Source: CAD feature listing. Evaluate the final solid. Frame: model axes, mm. Coordinates: 2 decimals unless noted, no trailing zeros. Write each loop counter-clockwise with the first axis right and the second up, starting at its lowest first coordinate (ties: lowest second). Pieces come first, ordered by that corner, then holes. Notation, with made-up numbers: M -20.5,-21 L 6.5,-21 A23 cw 6.5,12 Z; hole C -28,55 d7. An arc over 180 degrees is marked long. One line per item, written item: value. Start each with the question number.
Item 1: Ray query, L1, parallel to Z at x = 80, y = 1.75 (3 decimals); L2, parallel to X at y = 1, z = -0.25; L3, parallel to X at y = 2.35, z = 10. Return the intervals inside material, ascending. Write a range as from..to.
Item 2: Cut plane C-C, the plane y = 0.45. State how many separate pieces and enclosed holes the cut face has, then the cut area to 3 significant figures.
Item 3: Cut plane B-B, the plane x = 0. Output: boundary loops of the cut face in (y, z) (3 decimals), then the cut area to 4 significant figures.
Item 4: Cut plane A-A, the plane z = 0. Output: boundary loops of the cut face in (x, y) (3 decimals), then the cut area to 3 significant figures.
Item 5: Pin query (flat end, axial travel): P1, Ø3, axis at x = 80, z = 0, coming from the +Y side; P2, Ø1.5, axis at x = 66.5, y = 0.5, coming from the -Z side. Return the tip coordinate at first contact, or that it passes through.
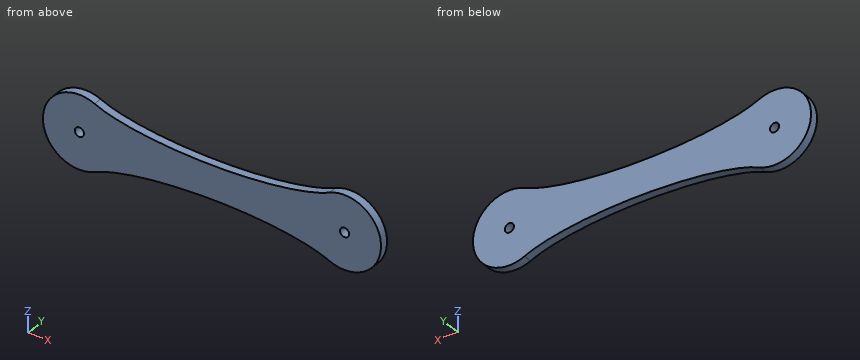
```python
from build123d import *

# Parameters (mm, degrees)
BOSS_EXTRUDE1_DEPTH = 2.6
CUT_EXTRUDE1_REACH  = 93.699
SKETCH3_R           = 1.375


with BuildPart() as part:
    # Sketch1 → Boss-Extrude1 (new body)
    with BuildSketch(Plane(origin=(0, 0, 0), x_dir=(1, 0, 0), z_dir=(0, 1, 0))):
        with BuildLine():
            ThreePointArc((4.582575695, 10), (-11, 0), (4.582575695, -10))
            add(Edge.make_bspline(
                [(4.582575695, -10), (11.56314995, -6.801099008), (40.099315353, -3.216443036), (68.360107676, -6.765931234), (75.417424305, -10)],
                knots=[0, 0, 0, 0, 0.499463492, 1, 1, 1, 1], degree=3))
            ThreePointArc((75.417424305, -10), (91, 0), (75.417424305, 10))
            add(Edge.make_bspline(
                [(4.582575695, 10), (11.56314995, 6.801099008), (40.099315353, 3.216443036), (68.360107676, 6.765931234), (75.417424305, 10)],
                knots=[0, 0, 0, 0, 0.499463492, 1, 1, 1, 1], degree=3))
        make_face()
    extrude(amount=BOSS_EXTRUDE1_DEPTH)

    # Sketch3 → Cut-Extrude1 (cut, up to next)
    with BuildSketch(Plane(origin=(0, 2.6, 0), x_dir=(1, 0, 0), z_dir=(0, 1, 0)), mode=Mode.PRIVATE) as cut_extrude1_sk1:
        with Locations(Location((0, 0, 0), (0, 0, 270))):
            Circle(SKETCH3_R)
    cut_extrude1_tool1 = extrude(cut_extrude1_sk1.sketch, amount=-CUT_EXTRUDE1_REACH, mode=Mode.PRIVATE) & part.part
    # Sketch3 → Cut-Extrude1 (cut, up to next)
    with BuildSketch(Plane(origin=(0, 2.6, 0), x_dir=(1, 0, 0), z_dir=(0, 1, 0)), mode=Mode.PRIVATE) as cut_extrude1_sk2:
        with Locations(Location((80, 0, 0), (0, 0, 270))):
            Circle(SKETCH3_R)
    cut_extrude1_tool2 = extrude(cut_extrude1_sk2.sketch, amount=-CUT_EXTRUDE1_REACH, mode=Mode.PRIVATE) & part.part
    add(cut_extrude1_tool1.solids().sort_by_distance((0, 2.6, 0))[0], mode=Mode.SUBTRACT)
    add(cut_extrude1_tool2.solids().sort_by_distance((80, 2.6, 0))[0], mode=Mode.SUBTRACT)


solid = part.part
```
From the geometry:
1. L1: z = -11..-1.375, 1.375..11
1. L2: x = -11..-1.35, 1.35..78.65, 81.35..91
1. L3: x = -4.58..4.58, 75.42..84.58
2. separate pieces: 1
2. enclosed holes: 2
2. area: 1,470 mm²
3. outline: M 0,-11 L 2.6,-11 L 2.6,-1.375 L 0,-1.375 Z; M 0,1.375 L 2.6,1.375 L 2.6,11 L 0,11 Z
3. area: 50.05 mm²
4. outline: M -11,0 L -1.375,0 L -1.375,2.6 L -11,2.6 Z; M 1.375,0 L 78.625,0 L 78.625,2.6 L 1.375,2.6 Z; M 81.375,0 L 91,0 L 91,2.6 L 81.375,2.6 Z
4. area: 251 mm²
5. P1: stops at y = 2.6
5. P2: stops at z = -7.47
